Build history of the part. All positions in model axes, mm. A direction names the side the tool comes from. Coordinates: 2 decimals unless noted, no trailing zeros. Order: outer loops, then holes, each group sorted by start corner. A loop starts at its lowest first (then second) coordinate and runs counter-clockwise, first axis right, second up. Notation, with made-up numbers: (-9.5, 62.25) - (0.5, 62.25) arc R20 ccw to (0.5, 98.25) - close; hole circle Ø5 at (39.25, -39). An arc over 180 degrees is marked (long way). Return JSON: item names as keys, results as strings.
from build123d import *

# Parameters (mm, degrees)
F0_W      = 65.024
F0_H      = 84.074
F1_DEPTH  = 35.052
F3_DEPTH  = 127
F4_W      = 72.461889
F4_H      = 59.973377
F5_DEPTH  = 127
F7_DEPTH  = 127
F9_DEPTH  = 127
F10_R     = 12.7
F11_DEPTH = 25.4
F12_R     = 8.001
F13_DEPTH = 65.025


with BuildPart() as f1:
    # F0 (on Right) → F1 (new body, symmetric)
    with BuildSketch(Plane.YZ):
        Rectangle(F0_W, F0_H)
    extrude(amount=F1_DEPTH, both=True)

    # F2 (on Front) → F3 (cut, symmetric)
    with BuildSketch(Plane.XZ):
        Polygon((-12.7, -3.937), (-44.45, -3.937), (-44.45, -67.437), (-12.7, -67.437), (-12.7, -21.463), (-7.112, -21.463), (-7.112, -16.637), (-12.7, -16.637), align=None)
        Polygon((44.45, -3.937), (12.7, -3.937), (12.7, -16.637), (7.112, -16.637), (7.112, -21.463), (12.7, -21.463), (12.7, -67.437), (44.45, -67.437), align=None)
    extrude(amount=F3_DEPTH, both=True, mode=Mode.SUBTRACT)

    # F4 (on Right) → F5 (cut, symmetric)
    with BuildSketch(Plane.YZ):
        with Locations((43.342944, 23.001689)):
            Rectangle(F4_W, F4_H)
    extrude(amount=F5_DEPTH, both=True, mode=Mode.SUBTRACT)

    # F6 (on face) → F7 (cut, symmetric)
    with BuildSketch(Plane.YZ.offset(12.7)):
        Polygon((22.86, 0.46973), (32.512, -42.037), (52.074212, -65.31479), (55.857351, 0.46973), align=None)
    extrude(amount=F7_DEPTH, both=True, mode=Mode.SUBTRACT)

    # F8 (on Right) → F9 (cut, symmetric)
    with BuildSketch(Plane.YZ):
        with BuildLine():
            ThreePointArc((-27.939918, 15.188745), (-17.613927, 39.957944), (7.20457, 50.164878))
            Line((7.20457, 50.164878), (-34.922153, 66.136815))
            Line((-34.922153, 66.136815), (-47.838565, 20.211793))
            Line((-47.838565, 20.211793), (-47.838565, 15.188745))
            Line((-47.838565, 15.188745), (-27.939918, 15.188745))
        make_face()
    extrude(amount=F9_DEPTH, both=True, mode=Mode.SUBTRACT)

    # F10 (on face) → F11 (join)
    with BuildSketch(Plane.XZ.offset(32.512)):
        with Locations((0, 15.113)):
            Circle(F10_R)
    extrude(amount=-F11_DEPTH)

    # F12 (on face) → F13 (cut, through all)
    with BuildSketch(Plane.XZ.offset(32.512)):
        with Locations((0, 15.113)):
            Circle(F12_R)
    extrude(amount=-F13_DEPTH, mode=Mode.SUBTRACT)


solid = f1.part
1. Cut at D-D on z = -29. Give the cut face in (x, y), plus the area to 3 significant figures.
Check values:
{"outline": "(-12.7, -32.51) - (12.7, -32.51) - (12.7, 29.55) - (-12.7, 29.55) - close", "area": "1,580 mm²"}
2. Cut at A-A on x = 0. Give the cut face in (y, z) (3 decimals).
Check values:
{"outline": "(-32.512, -42.037) - (32.512, -42.037) - (24.553, -6.985) - (7.112, -6.985) - (7.112, 7.112) - (-32.512, 7.112) - close; (-32.512, 23.114) - (7.112, 23.114) - (7.112, 42.037) - (-15.332, 42.037) arc R35.052 ccw to (-25.558, 27.813) - (-32.512, 27.813) - close"}
3. Drop flat-ended pins along their axis: pin 1 (10 mm diameter, centred on x = -11.5, z = 33, fed in from -Y); pin 2 (6.5 mm diameter, centred on y = 6.5, z = -12.5, fed in from -X); pin 3 (18.5 mm diameter, centred on x = 0, z = 15.113, fed in from +Y). Give the stop position or say it passes through.
Check values:
{"pin 1": "y = -25.49", "pin 2": "x = -12.7", "pin 3": "y = 7.11"}
4. Probe L1, parallel to Z at x = 0, y = -6; L2, parallel to X at y = 26, z = -36; L3, parallel to Y at x = -1, z = -6. List the from-to ranges inside material, lowest first.
Check values:
{"L1": "-42.04 to 7.11, 23.11 to 42.04", "L2": "-12.7 to 12.7", "L3": "-32.51 to 7.11"}
5. Mould opens along Z. For faces 4 (the flat face through (0, 0, -42.037)), 5 (the flat face through (0, -4, 42.037)), 6 (the cylindrical face through (-1.73, -12.98, 7.3)) say: pulls with the +Z half, pulls with the -Z half, needs draft (parallel to the pull), parting line crosses it, or undercut.
Check values:
{"face 4": "pulls with the -Z half", "face 5": "pulls with the +Z half", "face 6": "undercut"}
6. Tool access for faces 1 (the flat face through (-24, -30, 15.189)), 2 (the flat face through (10, -3, -16.637)), 3 (the flat face through (24, -30, 15.189)): list every direction of +Z, -Z, +X, -X, +Y, -Y with a clear straight run to the whole face (end or side of a thin tool).
Check values:
{"face 1": "+Z, -X, -Y", "face 2": "+X, +Y, -Y", "face 3": "+Z, +X, -Y"}
7. Cut at B-B on z = 13.5. Give the cut face in (x, y), plus the area to 3 significant figures.
Check values:
{"outline": "(-35.05, -32.51) - (-7.84, -32.51) - (-7.84, 7.11) - (-35.05, 7.11) - close; (7.84, -32.51) - (35.05, -32.51) - (35.05, 7.11) - (7.84, 7.11) - close", "area": "2,160 mm²"}
8. Cut at C-C on z = 3. Give the cut face in (x, y).
Check values:
{"outline": "(-35.05, -32.51) - (35.05, -32.51) - (35.05, 7.11) - (-35.05, 7.11) - close"}
